The listing builds one solid part. Answer for the finished solid, in the listing's coordinates (mm). Face numbers are marked on the shaded views. Give positions to 0.01 mm unless a question says otherwise; leave off trailing zeros. Order: outer loops, then holes, each group sorted by start corner. A loop starts at its lowest first (then second) coordinate and runs counter-clockwise, first axis right, second up.
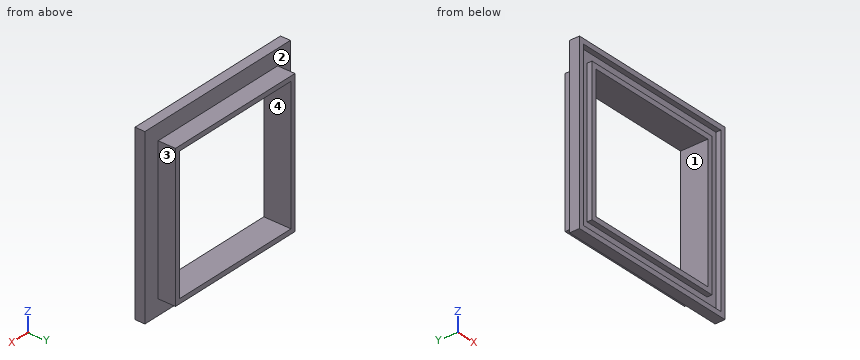
```python
from build123d import *

# Parameters (mm, degrees)
F0_W        = 70
F0_H        = 70
F0_W_2      = 64.5
F0_H_2      = 64.5
F0_W_3      = 57.5
F0_H_3      = 57.5
F0_W_4      = 53.7
F0_H_4      = 53.7
F1_DEPTH    = 11
F2_DEPTH    = 7
F3_T        = 2
F3_T3_DEPTH = 61.5
F3_T5_DEPTH = 61.5
F3_T7_DEPTH = 15


# Not quite as in the source:
# - a shell that OpenCascade refuses in one call is made with other operations: the cavity is built on its own and cut out


with BuildPart() as f1:
    # F0 (on Front) → F1 (new body)
    with BuildSketch(Plane.XZ):
        with Locations((35, 35)):
            Rectangle(F0_W, F0_H)
        with Locations((35, 35)):
            Rectangle(F0_W_2, F0_H_2, mode=Mode.SUBTRACT)
        with Locations((35, 35)):
            Rectangle(F0_W_2, F0_H_2)
        with Locations((34.9, 34.9)):
            Rectangle(F0_W_3, F0_H_3, mode=Mode.SUBTRACT)
        with Locations((34.9, 34.9)):
            Rectangle(F0_W_3, F0_H_3)
        with Locations((34.9, 34.9)):
            Rectangle(F0_W_4, F0_H_4, mode=Mode.SUBTRACT)
    extrude(amount=F1_DEPTH)

    # F0 (on Front) → F2 (cut)
    with BuildSketch(Plane.XZ):
        with Locations((35, 35)):
            Rectangle(F0_W, F0_H)
        with Locations((35, 35)):
            Rectangle(F0_W_2, F0_H_2, mode=Mode.SUBTRACT)
        with Locations((35, 35)):
            Rectangle(F0_W_2, F0_H_2)
        with Locations((34.9, 34.9)):
            Rectangle(F0_W_3, F0_H_3, mode=Mode.SUBTRACT)
    extrude(amount=F2_DEPTH, mode=Mode.SUBTRACT)

    # F3: shell of thickness 2, made by hand


with BuildPart() as f3_core1:
    # F3_t2: copy of F1
    add(f1.part)

    # the walls: a layer under each face that stays
    f3_faces = [f3_core1.faces().sort_by_distance(p)[0] for p in [
        (0, -9, 35),
        (5, -7, 5),
        (35, -9, 0),
        (35, -9, 70),
        (70, -9, 35),
        (63.65, -3.5, 34.9),
        (34.9, -3.5, 6.15),
        (6.15, -3.5, 34.9),
        (34.9, -3.5, 63.65),
        (34.9, -5.5, 8.05),
        (8.05, -5.5, 34.9),
        (34.9, -5.5, 61.75),
        (61.75, -5.5, 34.9),
        (7.946875, 0, 40.2240740741),
    ]]
    thicken(f3_faces, amount=-F3_T, mode=Mode.SUBTRACT)

    # F3_s4 → F3_t3 (cut)
    with BuildSketch(Plane.XY.offset(4.15)):
        Polygon((63.67, -6.98), (63.65, -9), (61.65, -9), (61.65, -7), align=None)
        Polygon((6.13, -6.98), (6.15, -9), (8.15, -9), (8.15, -7), align=None)
    extrude(amount=F3_T3_DEPTH, mode=Mode.SUBTRACT)

    # F3_s6 → F3_t5 (cut)
    with BuildSketch(Plane.YZ.offset(4.15)):
        Polygon((-6.98, 6.13), (-9, 6.15), (-9, 8.15), (-7, 8.15), align=None)
        Polygon((-6.98, 63.67), (-9, 63.65), (-9, 61.65), (-7, 61.65), align=None)
    extrude(amount=F3_T5_DEPTH, mode=Mode.SUBTRACT)

    # F3_s8 → F3_t7 (cut)
    with BuildSketch(Plane.XZ.offset(-2)):
        Polygon((61.73, 8.07), (61.75, 6.05), (63.75, 6.05), (63.75, 8.05), align=None)
        Polygon((8.07, 8.07), (8.05, 6.05), (6.05, 6.05), (6.05, 8.05), align=None)
        Polygon((8.07, 61.73), (6.05, 61.75), (6.05, 63.75), (8.05, 63.75), align=None)
        Polygon((61.73, 61.73), (61.75, 63.75), (63.75, 63.75), (63.75, 61.75), align=None)
    extrude(amount=F3_T7_DEPTH, mode=Mode.SUBTRACT)


with BuildPart() as f1_1:
    add(f1.part)

    # what is left inside the walls is the cavity
    f3_cavity = [f3_core1.part.solids().sort_by_distance(p)[0] for p in [
        (39.125, -9.02, 4.444444),
    ]]
    add(f3_cavity, mode=Mode.SUBTRACT)


solid = f1_1.part
```
1) Find section A-A (z = 49). Write down the section's boundary in (x, y).
Geometry says:
outline: (0, -11) - (2, -11) - (2, -9) - (6.05, -9) - (6.05, -11) - (8.05, -11) - (8.05, 0) - (6.15, 0) - (6.15, -7) - (0, -7) - close; (61.75, -11) - (63.75, -11) - (63.75, -9) - (68, -9) - (68, -11) - (70, -11) - (70, -7) - (63.65, -7) - (63.65, 0) - (61.75, 0) - close
2) Find section B-B (y = -10). Write down the section's boundary in (x, z), then the cut area to 3 significant figures.
Geometry says:
outline: (0, 0) - (70, 0) - (70, 70) - (0, 70) - close; (6.05, 6.05) - (63.75, 6.05) - (63.75, 63.75) - (6.05, 63.75) - close; hole (2, 2) - (68, 2) - (68, 68) - (2, 68) - close; hole (8.05, 8.05) - (61.75, 8.05) - (61.75, 61.75) - (8.05, 61.75) - close
area: 990 mm2
3) Given P1, Ø2, axis at x = 37, y = -9.5, coming from the -Z side; P2, Ø21, axis at x = 42.5, z = 19.5, coming from the +Y side; P3, Ø5, axis at x = 36.5, y = -4, coming from the -Z side; P4, Ø3.5, axis at y = -5, z = 39.5, coming from the +X side, each flat-ended and moving along its own axis, determine where each tip first touches the part or whether it passes through.
Geometry says:
P1: stops at z = 0
P2: passes through
P3: stops at z = 6.15
P4: stops at x = 63.65
4) For a pull along X with two mould halves and no side action, classify the marked faces 1, 2, 3 and 4 as +X half, -X half, draft (parallel to the pull), parting line (faces both ways), or undercut.
Geometry says:
face 1: undercut
face 2: draft
face 3: +X half
face 4: undercut
5) Straight lines are drawn through the part: probe 1 along X at (y, z) = (-9.75, 47.5); probe 2 along Z at (x, y) = (62, -10.25); probe 3 along Z at (x, y) = (60.5, -7.75). For each, find the intervals that lie inside material, in ascending order.
Geometry says:
probe 1: x = 0 to 2, 6.05 to 8.05, 61.75 to 63.75, 68 to 70
probe 2: z = 0 to 2, 6.05 to 63.75, 68 to 70
probe 3: z = 0 to 8.05, 61.75 to 70
6) Find section C-C (x = 37). Write down the section's boundary in (y, z).
Geometry says:
outline: (-11, 0) - (-7, 0) - (-7, 6.15) - (0, 6.15) - (0, 8.05) - (-11, 8.05) - (-11, 6.05) - (-9, 6.05) - (-9, 2) - (-11, 2) - close; (-11, 61.75) - (0, 61.75) - (0, 63.65) - (-7, 63.65) - (-7, 70) - (-11, 70) - (-11, 68) - (-9, 68) - (-9, 63.75) - (-11, 63.75) - close
7) Find section D-D (y = -4). Write down the section's boundary in (x, z).
Geometry says:
outline: (6.15, 6.15) - (63.65, 6.15) - (63.65, 63.65) - (6.15, 63.65) - close; hole (8.05, 8.05) - (61.75, 8.05) - (61.75, 61.75) - (8.05, 61.75) - close
